Read the model definition and answer for the solid it produces. Units are mm, in the model's axes. A direction names the side the tool comes from. Give positions to 0.01 mm unless a question says otherwise; leave off trailing zeros. Write each loop counter-clockwise with the first axis right and the second up, starting at its lowest first coordinate (ties: lowest second). Pieces come first, ordered by that corner, then holes. Notation, with made-up numbers: (-32, 52) -> (1, 52) arc R24 cw to (1, 73) -> close; hole circle Ø9 at (27, 83). An arc over 180 degrees is marked (long way). Use a Markdown table: item, result.
from build123d import *

# Parameters (mm, degrees)
BOSS_EXTRUDE1_DEPTH      = 53
BOSS_EXTRUDE1_DEPTH_BACK = 53
FILLET1_R                = 13
SHELL1_T                 = -3
CUT_EXTRUDE1_DEPTH       = 155.32757377
CUT_EXTRUDE1_DEPTH_BACK  = 155.32757377
CUT_EXTRUDE2_START       = -22.145
CUT_EXTRUDE2_DEPTH       = 5
FILLET2_R                = 2
SKETCH4_R                = 1.7
CUT_EXTRUDE3_DEPTH       = 10
SKETCH5_R                = 1.7
CUT_EXTRUDE6_DEPTH       = 10


with BuildPart() as part:
    # Sketch1 → Boss-Extrude1 (new, two sides: drawn at the far end of the back side and taken through both)
    with BuildSketch(Plane(origin=(0, -21.232774713, 56.11), x_dir=(0, -1, 0), z_dir=(-1, 0, 0)).offset(-BOSS_EXTRUDE1_DEPTH_BACK)):
        with BuildLine():
            Line((-18.232774713, -124.11), (-18.232774713, 11.89))
            Line((-18.232774713, 11.89), (-81.232774713, 11.89))
            ThreePointArc((-81.232774713, 11.89), (-149.232774713, -56.11), (-81.232774713, -124.11))
            Line((-81.232774713, -124.11), (-18.232774713, -124.11))
        make_face()
    extrude(amount=BOSS_EXTRUDE1_DEPTH + BOSS_EXTRUDE1_DEPTH_BACK)

    # Fillet1
    fillet1_edges = [part.edges().sort_by_distance(p)[0] for p in [
        (53, 28.5, 68),
        (53, 128, 0),
        (53, 28.5, -68),
        (-53, 28.5, 68),
        (-53, 28.5, -68),
        (-53, 128, 0),
    ]]
    fillet(fillet1_edges, radius=FILLET1_R)

    # Shell1
    shell1_openings = [part.faces().sort_by_distance(p)[0] for p in [
        (0, -3, 0),
    ]]
    offset(amount=SHELL1_T, openings=shell1_openings, kind=Kind.INTERSECTION)

    # Sketch2 → Cut-Extrude1 (cut, two sides: drawn at the far end of the back side and taken through both)
    with BuildSketch(Plane(origin=(0, 0, 0), x_dir=(0, 0, -1), z_dir=(1, 0, 0)).offset(-CUT_EXTRUDE1_DEPTH_BACK)):
        with BuildLine():
            Line((-26.582377719, 66.605088553), (-50.782987187, 73.089622316))
            ThreePointArc((-50.782987187, 73.089622316), (-52.639593743, 74.549701775), (-52.864046055, 76.900965497))
            ThreePointArc((-52.864046055, 76.900965497), (0, 115.5), (52.864046055, 76.900965497))
            ThreePointArc((52.864046055, 76.900965497), (52.639593743, 74.549701775), (50.782987187, 73.089622316))
            Line((50.782987187, 73.089622316), (26.582377719, 66.605088553))
            ThreePointArc((26.582377719, 66.605088553), (24.425691005, 66.839228235), (22.990729248, 68.466189737))
            ThreePointArc((22.990729248, 68.466189737), (0, 84.5), (-22.990729248, 68.466189737))
            ThreePointArc((-22.990729248, 68.466189737), (-24.425691005, 66.839228235), (-26.582377719, 66.605088553))
        make_face()
    extrude(amount=CUT_EXTRUDE1_DEPTH + CUT_EXTRUDE1_DEPTH_BACK, mode=Mode.SUBTRACT)

    # Sketch3 → Cut-Extrude2 (cut, symmetric)
    with BuildSketch(Plane(origin=(0, 0, 0), x_dir=(0, 0, -1), z_dir=(1, 0, 0)).offset(CUT_EXTRUDE2_START)):
        with BuildLine():
            Line((0, 60), (98.480775301, 77.364817767))
            ThreePointArc((98.480775301, 77.364817767), (0, 160), (-98.480775301, 77.364817767))
            Line((-98.480775301, 77.364817767), (0, 60))
        make_face()
    cut_extrude2 = extrude(amount=CUT_EXTRUDE2_DEPTH, both=True, mode=Mode.SUBTRACT)

    # Mirror1: Cut-Extrude2 across plane
    add(cut_extrude2.mirror(Plane(origin=(0, 0, 0), x_dir=(0, 0, 1), z_dir=(1, 0, 0))), mode=Mode.SUBTRACT)

    # Fillet2
    fillet2_edges = [part.edges().sort_by_distance(p)[0] for p in [
        (-17.145, 71.547603815, 65.489715575),
        (-17.145, 71.547603815, -65.489715575),
        (-27.145, 71.547603815, -65.489715575),
        (-27.145, 71.547603815, 65.489715575),
        (27.145, 71.547603815, 65.489715575),
        (27.145, 71.547603815, -65.489715575),
        (17.145, 71.547603815, -65.489715575),
        (17.145, 71.547603815, 65.489715575),
    ]]
    fillet(fillet2_edges, radius=FILLET2_R)

    # Sketch4 → Cut-Extrude3 (cut)
    with BuildSketch(Plane.XY.offset(68)):
        with Locations((0, 5)):
            Circle(SKETCH4_R)
    extrude(amount=-CUT_EXTRUDE3_DEPTH, mode=Mode.SUBTRACT)

    # Sketch5 → Cut-Extrude6 (cut)
    with BuildSketch(Plane(origin=(0, 0, -68), x_dir=(-1, 0, 0), z_dir=(0, 0, -1))):
        with Locations((25, 5)):
            Circle(SKETCH5_R)
        with Locations((-25, 5)):
            Circle(SKETCH5_R)
    extrude(amount=-CUT_EXTRUDE6_DEPTH, mode=Mode.SUBTRACT)


solid = part.part
Item 1: For a pull along X with two mould halves and no side action, classify faces 5 (the face through (53, 32, 1)), 6 (the face through (46.99, 28.06, -62.15)), 7 (the face through (-51.521, 69.893, -38.852)) as +X half, -X half, draft (parallel to the pull), parting line (faces both ways), or undercut.
Return value:
| item | result |
|---|---|
| face 5 | +X half |
| face 6 | undercut |
| face 7 | draft |
Item 2: A tool of negligible diameter and unlimited length cuts with its end or side. For faces 1 (the face through (-0.37, 3.34, 66.52)), 2 (the face through (-27.145, 125, -5)), 3 (the face through (-51.51, 115.49, 0.98)), 4 (the face through (1, 28, 65)), from which of +Z, -Z, +X, -X, +Y, -Y can it reach the whole face along a straight path? Write none if from no direction.
Return value:
| item | result |
|---|---|
| face 1 | +Z |
| face 2 | +Z, -Z, +Y |
| face 3 | +X, -X |
| face 4 | -Y |
Item 3: A cutting plane is placed at A-A (x = 8). Give the vertices of the cut face in (y, z), then the cut area to 3 significant figures.
Return value:
| item | result |
|---|---|
| outline | (-3, -68) -> (60, -68) arc R68 ccw to (60, 68) -> (-3, 68) -> (-3, 65) -> (60, 65) arc R65 cw to (60, -65) -> (-3, -65) -> close |
| area | 1,000 mm^2 |
Item 4: A cutting plane is placed at C-C (z = 9). Count the separate pieces of the cut face and the enclosed holes in it, then the cut area to 3 significant figures.
Return value:
| item | result |
|---|---|
| separate pieces | 5 |
| enclosed holes | 0 |
| area | 803 mm^2 |
Item 5: Straight lines are drawn through the part: line 1 along Z through (x, y) = (-27, 30); line 2 along X through (y, z) = (15.5, 39.5); line 3 along Z through (x, y) = (-44.5, 10). For each, find the intervals that lie inside material, in ascending order. Write a range as [from, to].
Return value:
| item | result |
|---|---|
| line 1 | [-68, -65], [65, 68] |
| line 2 | [-53, -50], [50, 53] |
| line 3 | [-67.2, -63.93], [63.93, 67.2] |
Item 6: A cutting plane is placed at D-D (x = 46). Give the vertices of the cut face in (y, z).
Return value:
| item | result |
|---|---|
| outline | (-3, -66.53) -> (60, -66.53) arc R66.53 ccw to (60, 66.53) -> (-3, 66.53) -> (-3, 63) -> (60, 63) arc R63 cw to (60, -63) -> (-3, -63) -> close |
Item 7: Each of these flat-tipped pins is pushed along its axis until it touches: P1, Ø6, axis at x = -21.5, z = -0.5, coming from the -Y side; P2, Ø2, axis at x = 5, z = -12, coming from the +Y side; P3, Ø16.5, axis at y = 99.5, z = -26.5, coming from the -X side; P4, Ø5, axis at x = -5.5, z = -39.5, coming from the +Y side. Where does it stop, or does it pass through?
Return value:
| item | result |
|---|---|
| P1 | through |
| P2 | y = 127.1 |
| P3 | x = -52.99 |
| P4 | y = 117.05 |
Item 8: A cutting plane is placed at B-B (y = 55). Give the vertices of the cut face in (x, z), then the cut area to 3 significant figures.
Return value:
| item | result |
|---|---|
| outline | (-53, -55) arc R13 ccw to (-40, -68) -> (40, -68) arc R13 ccw to (53, -55) -> (53, 55) arc R13 ccw to (40, 68) -> (-40, 68) arc R13 ccw to (-53, 55) -> close; hole (-50, -55) arc R10 ccw to (-40, -65) -> (40, -65) arc R10 ccw to (50, -55) -> (50, 55) arc R10 ccw to (40, 65) -> (-40, 65) arc R10 ccw to (-50, 55) -> close |
| area | 1,360 mm^2 |
